Drawing for the job (mm, zero at the part's lowest x, y, z). Give positions to 0.01 mm unless a question says otherwise; leave off trailing zeros. Write each loop counter-clockwise with the first axis right and the second up, starting at its lowest first coordinate (ties: lowest second). Pieces come first, ordered by that corner, then holes. Notation, with made-up numbers: M 71,-29 L 96,-29 A20 ccw 96,-1 Z; hole C 62.5,11.5 d1. An arc over 180 degrees is marked long. Use a Markdown table: item, result. Add a question column.
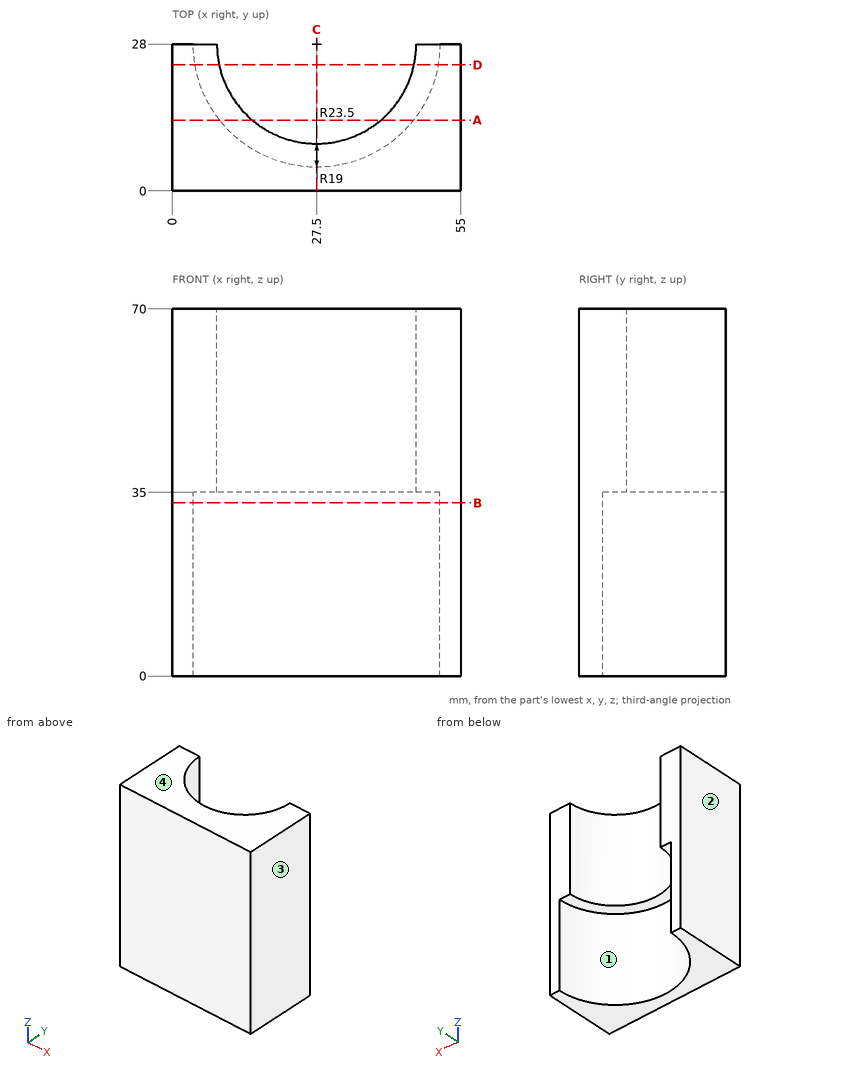
1. Cut at D-D (y = 24). Write the cut outline in (x, z).
2. Drill centre lines: probe 1 along X at (y, z) = (11.25, 16); probe 2 along X at (y, z) = (23, 28); probe 3 along Y at (x, z) = (27, 8). Where is each one in solid material? Low to high. Write a range as [from, to].
3. Cut at A-A (y = 13.5). Write the cut outline in (x, z), then the cut area to 3 significant figures.
4. Flat gauge pin, fed straight in: pin 1 (11.5 mm diameter, centred on x = 18.5, y = 18.5, fed in from -Z). Where does the tip first touch, or does it go through?
5. Cut at B-B (z = 33). Write the cut outline in (x, y), then the cut area to 3 significant figures.
6. Cut at C-C (x = 27.5). Write the cut outline in (y, z), then the cut area to 4 significant figures.
7. Mould opens along X. For the marked faces 1, 2, 3 and 4 say: released by +X, released by -X, zero draft, split by the parting line, or undercut.
A:
| question | item | result |
|---|---|---|
| 1 | outline | M 0,0 L 4.34,0 L 4.34,35 L 8.93,35 L 8.93,70 L 0,70 Z; M 46.07,35 L 50.66,35 L 50.66,0 L 55,0 L 55,70 L 46.07,70 Z |
| 2 | probe 1 | x = [0, 11.02], [43.98, 55] |
| 2 | probe 2 | x = [0, 4.54], [50.46, 55] |
| 2 | probe 3 | y = [0, 4.51] |
| 3 | outline | M 0,0 L 9.01,0 L 9.01,35 L 15.22,35 L 15.22,70 L 0,70 Z; M 39.78,35 L 45.99,35 L 45.99,0 L 55,0 L 55,70 L 39.78,70 Z |
| 3 | area | 1,700 mm² |
| 4 | pin 1 | passes through |
| 5 | outline | M 0,0 L 55,0 L 55,28 L 51,28 A23.5 cw 4,28 L 0,28 Z |
| 5 | area | 673 mm² |
| 6 | outline | M 0,0 L 4.5,0 L 4.5,35 L 9,35 L 9,70 L 0,70 Z |
| 6 | area | 472.5 mm² |
| 7 | face 1 | undercut |
| 7 | face 2 | released by -X |
| 7 | face 3 | released by +X |
| 7 | face 4 | zero draft |
